Verification items for this drawing (mm, ordinates from the low corner). A direction names the side the tool comes from. Coordinates: 2 decimals unless noted, no trailing zeros. Write each loop counter-clockwise with the first axis right and the second up, starting at its lowest first coordinate (ties: lowest second). Pieces come first, ordered by that corner, then holes. Notation, with made-up numbers: (58.25, 37.25) -> (78.25, 37.25) arc R7 cw to (78.25, 46.25) -> close; hole circle Ø8 at (55.25, 41). An arc over 180 degrees is marked (long way). Use CSV: the item, a comma, the result in double quotes.
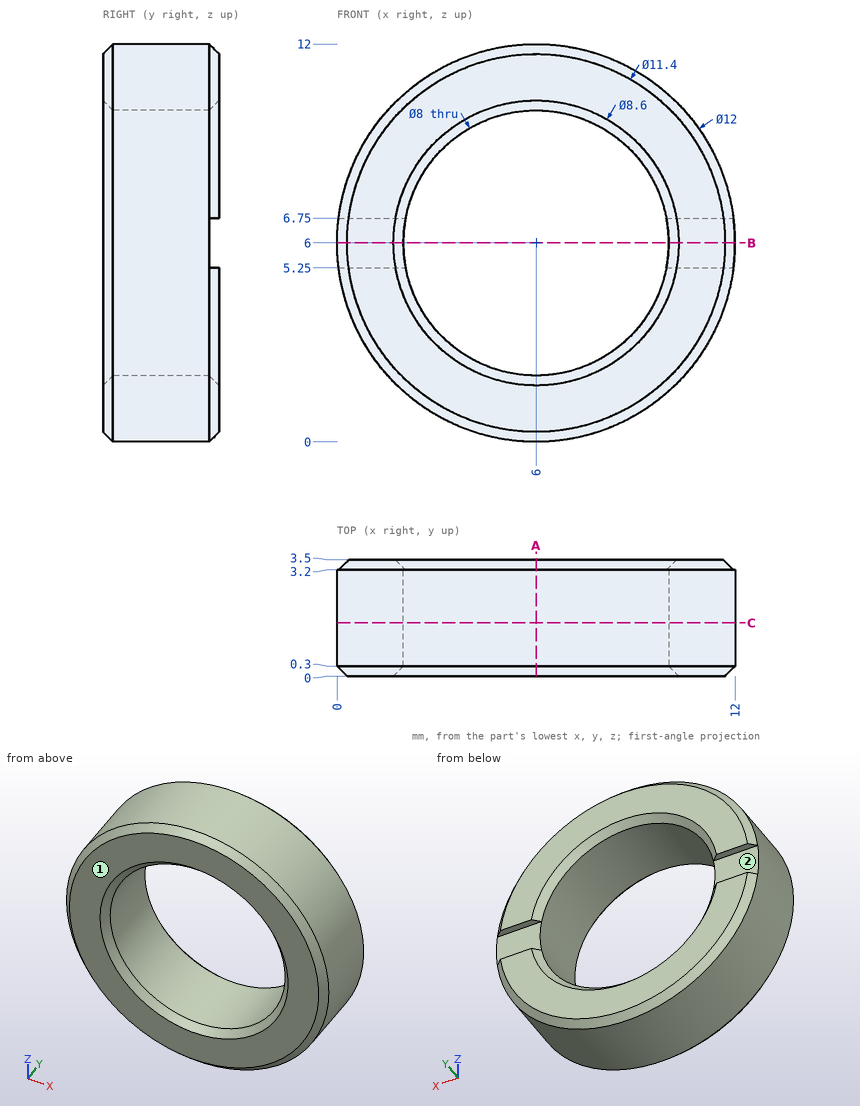
1) Cross-section at B-B (z = 6). Record the boundary of the cut face in (x, y), plus the area to 3 significant figures.
Return value:
outline,"(0, 0.3) -> (0.3, 0) -> (1.7, 0) -> (2, 0.3) -> (2, 3.2) -> (0, 3.2) -> close; (10, 0.3) -> (10.3, 0) -> (11.7, 0) -> (12, 0.3) -> (12, 3.2) -> (10, 3.2) -> close"
area,"12.6 mm2"
2) Set-up check for the marked faces 1 and 2: record each of +Z, -Z, +X, -X, +Y, -Y from which the full face is reachable in a straight line by a thin tool's end or side.
Return value:
face 1,"+Z, -Z, +X, -X, -Y"
face 2,"+X, -X, +Y"
3) Gauge pin test, flat ends, axial feed: pin 1 (0.8 mm diameter, centred on x = 1.5, z = 6, fed in from +Y); pin 2 (1.5 mm diameter, centred on y = 2.5, z = 9, fed in from +X); pin 3 (1.7 mm diameter, centred on x = 11.5, z = 5.5, fed in from +Y); pin 4 (6.5 mm diameter, centred on x = 6, z = 6, fed in from +Y). Record the tip position at first contact, or that the pin passes through.
Return value:
pin 1,"y = 3.2"
pin 2,"x = 11.56"
pin 3,"y = 3.5"
pin 4,"through"
4) Scan lines: L1, parallel to X at y = 2, z = 6; L2, parallel to X at y = 3, z = 6.75. Record each from-to range of solid material in increasing order.
Return value:
L1,"0 to 2, 10 to 12"
L2,"0.05 to 2.07, 9.93 to 11.95"
5) Cross-section at A-A (x = 6). Record the boundary of the cut face in (y, z), plus the area to 3 significant figures.
Return value:
outline,"(0, 0.3) -> (0.3, 0) -> (3.2, 0) -> (3.5, 0.3) -> (3.5, 1.7) -> (3.2, 2) -> (0.3, 2) -> (0, 1.7) -> close; (0, 10.3) -> (0.3, 10) -> (3.2, 10) -> (3.5, 10.3) -> (3.5, 11.7) -> (3.2, 12) -> (0.3, 12) -> (0, 11.7) -> close"
area,"13.6 mm2"
6) Cross-section at C-C (y = 1.6). Record the boundary of the cut face in (x, z).
Return value:
outline,"circle Ø12 at (6, 6); hole circle Ø8 at (6, 6)"
